CAD build for the part. Positions are in the model's coordinates, mm. A direction names the side the tool comes from. Round coordinates to 2 decimals unless told otherwise and drop trailing zeros. Loops run counter-clockwise (first coordinate to the right, second up) from the corner with the lowest first, then second, coordinate; pieces in that order, holes last. Notation, with made-up numbers: (0.25, -34.5) - (32.25, -34.5) arc R10 ccw to (32.25, -18.5) - close; hole circle Ø5 at (31.5, 86.5). An arc over 180 degrees is marked (long way). Use one line per item in the form item = value.
from build123d import *

# Parameters (mm, degrees)
F2_SIZE = 0.2
F3_R    = 1


with BuildPart() as f1:
    # F0 (on Top) → F1 (revolve)
    with BuildSketch(Plane.XY):
        Polygon((2.5, 6), (2.5, 0), (4, 0), (4, 7), (5.75, 7), (5.75, 7.4), (10.75, 7.4), (10.75, 9), (0, 9), (0, 6), align=None)
    revolve(axis=Axis((0, 4.843669, 0), (0, -1, 0)))

    # F2
    f2_edges = [f1.edges().sort_by_distance(p)[0] for p in [
        (-4, 0, 0),
    ]]
    chamfer(f2_edges, length=F2_SIZE)

    # F3
    f3_edges = [f1.edges().sort_by_distance(p)[0] for p in [
        (-10.75, 9, 0),
    ]]
    fillet(f3_edges, radius=F3_R)


solid = f1.part
1) Tool access for faces 1 (the cylindrical face through (-0.867, 3.648, -3.905)), 2 (the flat face through (0.9, 0, -2.5)): list every direction of +Z, -Z, +X, -X, +Y, -Y with a clear straight run to the whole face (end or side of a thin tool).
Report:
face_1 = -Y
face_2 = +Z, -Z, +X, -X, -Y
2) Slice it at B-B (y = 3). Write the cut outline in (x, z).
Report:
outline = circle Ø8 at (0, 0); hole circle Ø5 at (0, 0)
3) Flat gauge pins, fed straight in: pin 1 (5 mm diameter, centred on y = 1.5, z = -4.5, fed in from +X); pin 2 (4 mm diameter, centred on x = 0.5, y = 2.5, fed in from -Z). Where does each tip first touch, or does it go through?
Report:
pin_1 = 3.46
pin_2 = -4
4) Slice it at A-A (x = 0). Write the cut outline in (y, z).
Report:
outline = (0, -3.8) - (0.2, -4) - (7, -4) - (7, -5.75) - (7.4, -5.75) - (7.4, -10.75) - (8, -10.75) arc R1 ccw to (9, -9.75) - (9, 9.75) arc R1 ccw to (8, 10.75) - (7.4, 10.75) - (7.4, 5.75) - (7, 5.75) - (7, 4) - (0.2, 4) - (0, 3.8) - (0, 2.5) - (6, 2.5) - (6, -2.5) - (0, -2.5) - close
5) Two-plate mould, pull along Z, no slides. Class faces 3 (the flat face through (-5, 7.4, -5)), 4 (the cylindrical face through (-0.54, 2.96, -2.44)), 5 (the cylindrical face through (-1.4, 7.7, 10.66)): +Z half, -Z half, draft (parallel to the pull), parting line (faces both ways), or undercut.
Report:
face_3 = draft
face_4 = undercut
face_5 = parting line
6) Drill centre lines: probe 1 along Z at (x, y) = (0, 3.3); probe 2 along Y at (x, z) = (-5, 2); probe 3 along Y at (x, z) = (8.75, 0). Where is each one in solid material? Low to high.
Report:
probe_1 = -4 to -2.5, 2.5 to 4
probe_2 = 7 to 9
probe_3 = 7.4 to 9
7) Slice it at C-C (z = 0). Write the cut outline in (x, y).
Report:
outline = (-10.75, 7.4) - (-5.75, 7.4) - (-5.75, 7) - (-4, 7) - (-4, 0.2) - (-3.8, 0) - (-2.5, 0) - (-2.5, 6) - (2.5, 6) - (2.5, 0) - (3.8, 0) - (4, 0.2) - (4, 7) - (5.75, 7) - (5.75, 7.4) - (10.75, 7.4) - (10.75, 8) arc R1 ccw to (9.75, 9) - (-9.75, 9) arc R1 ccw to (-10.75, 8) - close
